```python
from build123d import *

# Parameters (mm, degrees)
SKETCH1_R            = 20
BOSS_EXTRUDE1_DEPTH  = 5.08
SKETCH2_R            = 9.525
BOSS_EXTRUDE2_DEPTH  = 12.7
M5_CLEARANCE_HOLE1_D = 5.5
CUT_EXTRUDE1_DEPTH   = 18.78
FILLET1_R            = 2.54


with BuildPart() as part:
    # Sketch1 → Boss-Extrude1 (new body)
    with BuildSketch(Plane.XY):
        Circle(SKETCH1_R)
    extrude(amount=BOSS_EXTRUDE1_DEPTH)

    # Sketch2 → Boss-Extrude2 (add)
    with BuildSketch(Plane.XY.offset(5.08)):
        Circle(SKETCH2_R)
    extrude(amount=BOSS_EXTRUDE2_DEPTH)

    # M5 Clearance Hole1 (through all)
    with Locations(Plane.XY.offset(5.08)):
        with Locations((0, 15.5), (13.423393759, -7.75), (-13.423393759, -7.75)):
            Hole(M5_CLEARANCE_HOLE1_D / 2)

    # Sketch5 → Cut-Extrude1 (cut, through all)
    with BuildSketch(Plane.XY.offset(17.78)):
        Polygon((3.666174209, 6.35), (-3.666174209, 6.35), (-7.332348419, 0), (-3.666174209, -6.35), (3.666174209, -6.35), (7.332348419, 0), align=None)
    extrude(amount=-CUT_EXTRUDE1_DEPTH, mode=Mode.SUBTRACT)

    # Fillet1
    fillet1_edges = [part.edges().sort_by_distance(p)[0] for p in [
        (-9.525, 0, 5.08),
    ]]
    fillet(fillet1_edges, radius=FILLET1_R)


solid = part.part
```
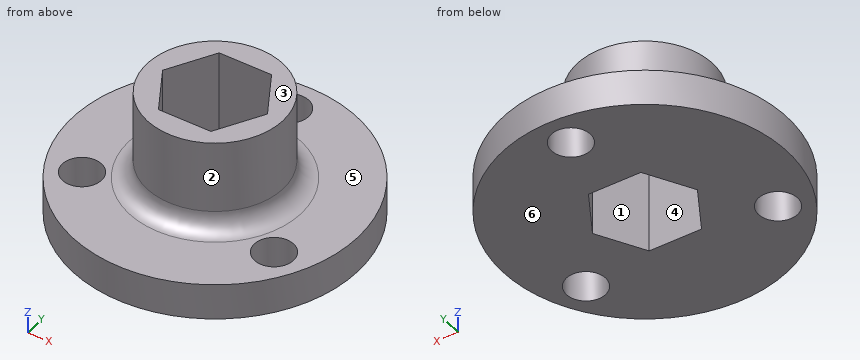
The model under review builds one solid part; all positions refer to its coordinate system, in mm. Face numbers are marked on the shaded views. A direction names the side the tool comes from. Coordinates: 2 decimals unless noted, no trailing zeros. Write each loop counter-clockwise with the first axis right and the second up, starting at its lowest first coordinate (ties: lowest second). Pieces come first, ordered by that corner, then holes. Notation, with made-up numbers: (75.5, -34) -> (107.5, -34) arc R10 cw to (107.5, -21) -> close; hole circle Ø1 at (-14.5, 50.5). An arc over 180 degrees is marked (long way). One line per item, written item: value. Start each with the question number.
Q1. The part is to be moulded in two halves that separate along Y. For the marked faces 1, 2 and 3, say which applies: +Y half, -Y half, draft (parallel to the pull), parting line (faces both ways), or undercut.
Q2. Add section C-C, the plane y = -10. Count the separate pieces of the cut face and the enclosed holes in it, then the cut area to 3 significant figures.
Q3. Add section A-A, the plane z = 8.25. Give the boundary of the cut face in (x, y) (3 decimals), then the cut area to 3 significant figures.
Q4. For the marked faces 4, 5 and 6, list the 3-axis set-ups (+Z, -Z, +X, -X, +Y, -Y) from which the entire face can be reached by the end or side of a thin tool; tool diameter is ignored.
Q5. Clearance check with flat-ended pins moving along their axes: P1, Ø6, axis at x = 1.5, z = 8.5, coming from the +Y side; P2, Ø4, axis at x = -10.5, z = 12, coming from the -Y side; P3, Ø4, axis at y = 1.5, z = 13.5, coming from the +X side (3 decimals). State where each tip first meets the part, or that it passes through.
Q6. To check wall thickness, follow probe 1 along Y at (x, z) = (0, 3.45); probe 2 along Y at (x, z) = (2.5, 5); probe 3 along Z at (x, y) = (14.5, -3). State the ranges of each line that lie inside material, in increasing order.
Q7. Add section B-B, the plane y = 15.5. Give the boundary of the cut face in (x, z), then the cut area to 3 significant figures.
Response:
1. face 1: undercut
1. face 2: parting line
1. face 3: draft
2. separate pieces: 3
2. enclosed holes: 0
2. area: 151 mm²
3. outline: circle Ø19.05 at (0, 0); hole (-7.332, 0) -> (-3.666, -6.35) -> (3.666, -6.35) -> (7.332, 0) -> (3.666, 6.35) -> (-3.666, 6.35) -> close
3. area: 145 mm²
4. face 4: +Z, -Z
4. face 5: +Z
4. face 6: -Z, +X, -X, +Y, -Y
5. P1: y = 10.58
5. P2: y = -4.3
5. P3: x = 9.525
6. probe 1: -20 to -6.35, 6.35 to 12.75, 18.25 to 20
6. probe 2: -19.84 to -6.35, 6.35 to 14.35, 16.65 to 19.84
6. probe 3: 0 to 5.08
7. outline: (-12.64, 0) -> (-2.75, 0) -> (-2.75, 5.08) -> (-12.64, 5.08) -> close; (2.75, 0) -> (12.64, 0) -> (12.64, 5.08) -> (2.75, 5.08) -> close
7. area: 100 mm²
